Read the model definition and answer for the solid it produces. Units are mm, in the model's axes. Face numbers are marked on the shaded views. Give positions to 0.01 mm unless a question says otherwise; leave off trailing zeros. Loops run counter-clockwise (first coordinate to the right, second up) from the corner with the lowest first, then second, coordinate; pieces in that order, holes last. Notation, with made-up numbers: (-37.5, 25.25) -> (2.5, 25.25) arc R18 cw to (2.5, 50.25) -> close; hole circle Ø7 at (79, 22). An arc over 180 degrees is marked (long way). Answer as CSV lines item,"result". Start each with the question number.
```python
from build123d import *

# Parameters (mm, degrees)
F0_R     = 91.6
F1_DEPTH = 6
F2_R     = 2
F3_T     = -1.6
F6_R     = 30
F7_DEPTH = 50
F8_R     = 26.5
F9_DEPTH = 56.001
F12_D    = 8.8


with BuildPart() as f1:
    # F0 (on Top) → F1 (new body)
    with BuildSketch(Plane.XY):
        Circle(F0_R)
    extrude(amount=F1_DEPTH)

    # F2
    f2_edges = [f1.edges().sort_by_distance(p)[0] for p in [
        (-91.6, 0, 6),
    ]]
    fillet(f2_edges, radius=F2_R)

    # F3
    f3_openings = [f1.faces().sort_by_distance(p)[0] for p in [
        (0, 0, 0),
    ]]
    offset(amount=F3_T, openings=f3_openings)


with BuildPart() as f5_1:
    # F5: copy of F1
    add(f1.part)


with BuildPart() as f7:
    # F6 (on face) → F7 (new body)
    with BuildSketch(Plane.XY.offset(6)):
        Circle(F6_R)
    extrude(amount=F7_DEPTH)

    # F8 (on face) → F9 (cut, through all)
    with BuildSketch(Plane.XY.offset(56)):
        Circle(F8_R)
    extrude(amount=-F9_DEPTH, mode=Mode.SUBTRACT)


with BuildPart() as f1_1:
    add(f1.part)

    # F12 (through all)
    with Locations(Plane.XY.offset(6)):
        with Locations((0, 0)):
            Hole(F12_D / 2)


solid = f1_1.part
```
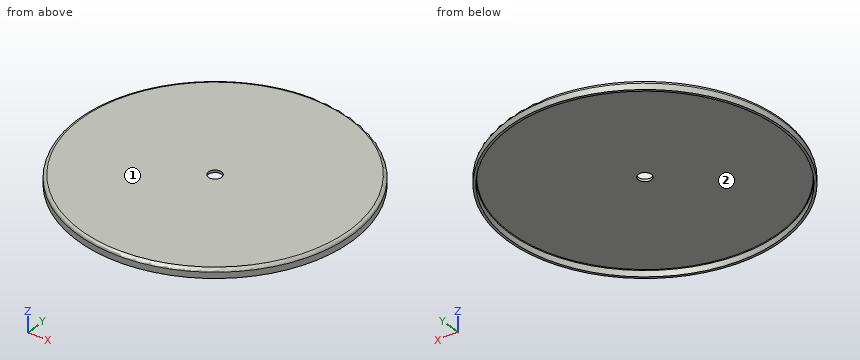
(1) Find the intervals of material crossed by line 1 along X through (y, z) = (-1, 3.7); line 2 along Y through (x, z) = (0, 0.85); line 3 along Z through (x, y) = (22, 63), in increasing order. Write a range as from..to.
(2) Find section C-C on z = 3. Write down the section's boundary in (x, y).
(3) The mould has two halves that part along Y. Classify the marked faces 1 and 2: pulls with the +Y half, pulls with the -Y half, needs draft (parallel to the pull), parting line crosses it, or undercut.
(4) Each of these flat-tipped pins is pushed along its axis until it touches: P1, Ø5, axis at x = -14, y = 26.5, coming from the -Z side; P2, Ø2, axis at x = -20.5, z = 1.5, coming from the +Y side; P3, Ø8, axis at x = 0, y = 0, coming from the -Z side; P4, Ø2, axis at x = 25.5, z = 1, coming from the +Y side. Where does it stop, or does it pass through?
(5) Find section A-A on y = 0. Write down the section's boundary in (x, z), then the cut area to 3 significant figures.
Answer block:
1,line 1,"x = -91.59..-89.99, 89.99..91.59"
1,line 2,"y = -91.6..-90, 90..91.6"
1,line 3,"z = 4.4..6"
2,outline,"circle Ø183.2 at (0, 0); hole circle Ø180 at (0, 0)"
3,face 1,"needs draft"
3,face 2,"undercut"
4,P1,"stops at z = 4.4"
4,P2,"stops at y = 89.5"
4,P3,"passes through"
4,P4,"stops at y = 88.26"
5,outline,"(-91.6, 0) -> (-90, 0) -> (-90, 4) arc R0.4 cw to (-89.6, 4.4) -> (-4.4, 4.4) -> (-4.4, 6) -> (-89.6, 6) arc R2 ccw to (-91.6, 4) -> close; (4.4, 4.4) -> (89.6, 4.4) arc R0.4 cw to (90, 4) -> (90, 0) -> (91.6, 0) -> (91.6, 4) arc R2 ccw to (89.6, 6) -> (4.4, 6) -> close"
5,area,"291 mm2"
